from build123d import *

# Parameters (mm, degrees)
ESQUISSE1_W             = 5
ESQUISSE1_H             = 150
ESQUISSE1_R             = 15
BASE_DEPTH              = 10
VIDE_VIS_DEPTH          = 127.219055614
VIDE_VIS_DEPTH_BACK     = 127.219055614
ESQUISSE5_R             = 2.5
ESQUISSE6_W             = 130
ESQUISSE6_H             = 150
ENL_V_MAT_EXTRU_6_DEPTH = 5
VIDE_TEST_DEPTH         = 118.100384286
ESQUISSE8_W             = 31.25
ESQUISSE8_H             = 6.85
BOSS_FERME_DEPTH        = 10
CONGE_TEST_R            = 1


with BuildPart() as part:
    # Esquisse1 → BASE (new body)
    with BuildSketch(Plane(origin=(0, 0, 0), x_dir=(1, 0, 0), z_dir=(0, 1, 0))):
        Polygon((-82.5, 82.5), (-82.5, 77.5), (-72.5, 77.5), (-72.5, 67.5), (-82.5, 67.5), (-82.5, -2.5), (-72.5, -2.5), (-72.5, -12.5), (-82.5, -12.5), (-82.5, -82.5), (82.5, -82.5), (82.5, -12.5), (72.5, -12.5), (72.5, -2.5), (82.5, -2.5), (82.5, 67.5), (72.5, 67.5), (72.5, 77.5), (82.5, 77.5), (82.5, 82.5), align=None)
        with BuildLine():
            ThreePointArc((-12.916666667, -10.915030923), (-10.627210874, -13.27000839), (-7.916666667, -15.124860621))
            Line((-7.916666667, -15.124860621), (-7.916666667, -75.648107225))
            Line((-7.916666667, -75.648107225), (-12.916666667, -75.648107225))
            Line((-12.916666667, -75.648107225), (-12.916666667, -10.915030923))
        make_face(mode=Mode.SUBTRACT)
        with Locations((-62.5, -0.648107225)):
            Rectangle(ESQUISSE1_W, ESQUISSE1_H, mode=Mode.SUBTRACT)
        with Locations((-52.083333333, -0.648107225)):
            Rectangle(ESQUISSE1_W, ESQUISSE1_H, mode=Mode.SUBTRACT)
        with Locations((-41.666666667, -0.648107225)):
            Rectangle(ESQUISSE1_W, ESQUISSE1_H, mode=Mode.SUBTRACT)
        with Locations((-31.25, -0.648107225)):
            Rectangle(ESQUISSE1_W, ESQUISSE1_H, mode=Mode.SUBTRACT)
        with Locations((-20.833333333, -0.648107225)):
            Rectangle(ESQUISSE1_W, ESQUISSE1_H, mode=Mode.SUBTRACT)
        with Locations(Location((0, -0.648107225, 0), (0, 0, 270))):
            Circle(ESQUISSE1_R, mode=Mode.SUBTRACT)
        with BuildLine():
            Line((-2.5, -75.648107225), (-2.5, -16.957613655))
            ThreePointArc((-2.5, -16.957613655), (0, -17.148107225), (2.5, -16.957613655))
            Line((2.5, -16.957613655), (2.5, -75.648107225))
            Line((2.5, -75.648107225), (-2.5, -75.648107225))
        make_face(mode=Mode.SUBTRACT)
        with BuildLine():
            Line((7.916666667, -75.648107225), (7.916666667, -15.124860621))
            ThreePointArc((7.916666667, -15.124860621), (10.627210874, -13.27000839), (12.916666667, -10.915030923))
            Line((12.916666667, -10.915030923), (12.916666667, -75.648107225))
            Line((12.916666667, -75.648107225), (7.916666667, -75.648107225))
        make_face(mode=Mode.SUBTRACT)
        with BuildLine():
            Line((-12.916666667, 9.618816473), (-12.916666667, 74.351892775))
            Line((-12.916666667, 74.351892775), (-7.916666667, 74.351892775))
            Line((-7.916666667, 74.351892775), (-7.916666667, 13.828646171))
            ThreePointArc((-7.916666667, 13.828646171), (-10.627210874, 11.973793941), (-12.916666667, 9.618816473))
        make_face(mode=Mode.SUBTRACT)
        with Locations((20.833333333, -0.648107225)):
            Rectangle(ESQUISSE1_W, ESQUISSE1_H, mode=Mode.SUBTRACT)
        with Locations((31.25, -0.648107225)):
            Rectangle(ESQUISSE1_W, ESQUISSE1_H, mode=Mode.SUBTRACT)
        with Locations((41.666666667, -0.648107225)):
            Rectangle(ESQUISSE1_W, ESQUISSE1_H, mode=Mode.SUBTRACT)
        with Locations((52.083333333, -0.648107225)):
            Rectangle(ESQUISSE1_W, ESQUISSE1_H, mode=Mode.SUBTRACT)
        with Locations((62.5, -0.648107225)):
            Rectangle(ESQUISSE1_W, ESQUISSE1_H, mode=Mode.SUBTRACT)
        with BuildLine():
            Line((-2.5, 15.661399205), (-2.5, 74.351892775))
            Line((-2.5, 74.351892775), (2.5, 74.351892775))
            Line((2.5, 74.351892775), (2.5, 15.661399205))
            ThreePointArc((2.5, 15.661399205), (0, 15.851892775), (-2.5, 15.661399205))
        make_face(mode=Mode.SUBTRACT)
        with BuildLine():
            Line((12.916666667, 74.351892775), (12.916666667, 9.618816473))
            ThreePointArc((12.916666667, 9.618816473), (10.627210874, 11.973793941), (7.916666667, 13.828646171))
            Line((7.916666667, 13.828646171), (7.916666667, 74.351892775))
            Line((7.916666667, 74.351892775), (12.916666667, 74.351892775))
        make_face(mode=Mode.SUBTRACT)
    extrude(amount=BASE_DEPTH)

    # Esquisse5 → VIDE VIS (cut, two sides: drawn at the far end of the back side and taken through both)
    with BuildSketch(Plane(origin=(0, 0, 12.5), x_dir=(-1, 0, 0), z_dir=(0, 0, -1)).offset(-VIDE_VIS_DEPTH_BACK)):
        with Locations((-77.5, 5)):
            Circle(ESQUISSE5_R)
        with Locations(Location((77.5, 5, 0), (0, 0, 180))):
            Circle(ESQUISSE5_R)
    extrude(amount=VIDE_VIS_DEPTH + VIDE_VIS_DEPTH_BACK, mode=Mode.SUBTRACT)

    # Esquisse6 → Enlèv. mat.-Extru.6 (cut)
    with BuildSketch(Plane.XZ):
        with Locations((0, 0.648107225)):
            Rectangle(ESQUISSE6_W, ESQUISSE6_H)
    extrude(amount=-ENL_V_MAT_EXTRU_6_DEPTH, mode=Mode.SUBTRACT)

    # Esquisse7 → VIDE TEST (cut, through all)
    with BuildSketch(Plane(origin=(0, 10, 0), x_dir=(1, 0, 0), z_dir=(0, 1, 0))):
        Polygon((-33.75, -25.416267648), (-33.75, -82.5), (82.5, -82.5), (82.5, 82.5), (-82.5, 82.5), (-82.5, -25.416267648), align=None)
    extrude(amount=-VIDE_TEST_DEPTH, mode=Mode.SUBTRACT)

    # Esquisse8 → BOSS FERME (add)
    with BuildSketch(Plane.XZ):
        with Locations((-49.375, 28.841267648)):
            Rectangle(ESQUISSE8_W, ESQUISSE8_H)
    extrude(amount=-BOSS_FERME_DEPTH)

    # CONGE TEST
    conge_test_edges = [part.edges().sort_by_distance(p)[0] for p in [
        (-54.583333333, 5, 53.957187436),
        (-49.583333333, 5, 53.957187436),
    ]]
    fillet(conge_test_edges, radius=CONGE_TEST_R)


solid = part.part
Can you work these out from the model? Positions are in its coordinate system, mm. A direction names the side the tool comes from. Round coordinates to 2 decimals unless told otherwise and drop trailing zeros. Write each loop counter-clockwise with the first axis right and the second up, starting at its lowest first coordinate (ties: lowest second). Pieces come first, ordered by that corner, then holes. Notation, with made-up numbers: (24, 45) -> (50, 45) arc R17 cw to (50, 78) -> close; hole circle Ø2 at (70, 51). An arc over 180 degrees is marked (long way). One line per question, with ' | ' between items. Start each with the question number.
1) Suppose I cut it at D-D on x = -41.5. Write out the boundary of the cut face in (y, z), then the cut area to 3 significant figures.
2) I'm going to push a flat-ended pin straight in: P1, Ø1.3, axis at x = -58, z = 59.5, coming from the -Y side. Where does the tip first touch, or does it pass through?
3) I need wall thicknesses on line 1 (X direction, y = 9.75, z = 75); line 2 (Z direction, x = -41, y = 6.75); line 3 (Y direction, x = -77.5, z = 58.5). Which ranges of each line are inside material? Lowest first, please. Write a range as [from, to].
4) Suppose I cut it at C-C on x = -57.5. Write out the boundary of the cut face in (y, z), then the cut area to 3 significant figures.
5) Suppose I cut it at A-A on x = -77.5. Write out the boundary of the cut face in (y, z).
6) On a 3-axis mill with a long thin cutter (end or side, diameter ignored), from which of +Z, -Z, +X, -X, +Y, -Y can I reach the whole of each face in a straight line? I mean faces 5 (the flat face through (-49.583, 8, 54)), 6 (the flat face through (-58, 5, 54)), 7 (the flat face through (-50, 5, 32.266)). Say none if no direction works.
7) If we mould it in two halves opening along Z, with no side actions, what happens to faces 1 (the flat face through (-58, 5, 82.5)), 2 (the flat face through (-36, 5, 54)), 3 (the flat face through (-58, 10, 54)), 4 (the flat face through (-58, 5, 25.416))? For each: released by +Z, released by -Z, zero draft, split by the parting line, or undercut.
8) Suppose I cut it at B-B on z = 48.5. Write out the boundary of the cut face in (x, y), then the cut area to 3 significant figures.
Return value:
1) outline: (0, 25.42) -> (10, 25.42) -> (10, 32.27) -> (0, 32.27) -> close; (0, 75.65) -> (10, 75.65) -> (10, 82.5) -> (0, 82.5) -> close | area: 137 mm2
2) P1: stops at y = 5
3) line 1: x = [-82.5, -65], [-60, -54.58], [-49.58, -44.17], [-39.17, -33.75] | line 2: z = [25.42, 32.27], [75.65, 82.5] | line 3: y = [0, 2.5], [7.5, 10]
4) outline: (0, 25.42) -> (10, 25.42) -> (10, 82.5) -> (0, 82.5) -> (0, 75.65) -> (5, 75.65) -> (5, 32.27) -> (0, 32.27) -> close | area: 354 mm2
5) outline: (0, 25.42) -> (2.5, 25.42) -> (2.5, 82.5) -> (0, 82.5) -> close; (7.5, 25.42) -> (10, 25.42) -> (10, 82.5) -> (7.5, 82.5) -> close
6) face 5: +Y, -Y | face 6: +X, -Y | face 7: -Y
7) face 1: released by +Z | face 2: undercut | face 3: zero draft | face 4: released by -Z
8) outline: (-82.5, 0) -> (-65, 0) -> (-65, 10) -> (-82.5, 10) -> close; (-60, 5) -> (-55.58, 5) arc R1 ccw to (-54.58, 6) -> (-54.58, 10) -> (-60, 10) -> close; (-49.58, 6) arc R1 ccw to (-48.58, 5) -> (-44.17, 5) -> (-44.17, 10) -> (-49.58, 10) -> close; (-39.17, 5) -> (-33.75, 5) -> (-33.75, 10) -> (-39.17, 10) -> close; hole circle Ø5 at (-77.5, 5) | area: 236 mm2
